```python
from build123d import *

# Parameters (mm, degrees)
F0_R      = 31.75
F1_DEPTH  = 101.6
F0_W      = 88.9
F0_H      = 6.35
F2_R      = 6.35
F3_SIZE   = 3.175
F6_DEPTH  = 88.9
F7_R      = 5.08
F8_W      = 12.7
F8_H      = 25.4
F9_DEPTH  = 88.9
F10_R     = 6.35
F11_R     = 9.525
F12_DEPTH = 6.35
F13_R     = 6.35
F14_DEPTH = 38.1


with BuildPart() as f1:
    # F0 (on Front) → F1 (new body)
    with BuildSketch(Plane.XZ):
        with Locations((0, 44.45)):
            Circle(F0_R)
    extrude(amount=-F1_DEPTH)

    # F2
    f2_edges = [f1.edges().sort_by_distance(p)[0] for p in [
        (-31.75, 0, 44.45),
        (-31.75, 101.6, 44.45),
    ]]
    fillet(f2_edges, radius=F2_R)

    # F5 (on offset) → F6 (join)
    with BuildSketch(Plane(origin=(0, 95.25, 0), x_dir=(-1, 0, 0), z_dir=(0, 1, 0))):
        Polygon((1.5875, 49.3358226153), (1.5875, 82.55), (-1.5875, 82.55), (-1.5875, 49.3358226153), (0, 47.1508163165), align=None)
        Polygon((21.1103036338, 76.2066565737), (1.5875, 49.3358226153), (1.5875, 46.6350062987), (4.1561289571, 47.4696044392), (23.6789325909, 74.3404383977), align=None)
        Polygon((1.5875, 46.6350062987), (1.5875, 49.3358226153), (0, 47.1508163165), (0.6063710429, 46.316218176), align=None)
        Polygon((0, 47.1508163165), (-1.5875, 49.3358226153), (-1.5875, 46.6350062987), (-0.6063710429, 46.316218176), align=None)
        Polygon((-1.5875, 46.6350062987), (-1.5875, 49.3358226153), (-21.1103036338, 76.2066565737), (-23.6789325909, 74.3404383977), (-4.1561289571, 47.4696044392), align=None)
        Polygon((4.1561289571, 47.4696044392), (1.5875, 46.6350062987), (1.5875, 45.6033862632), (2.5686289571, 45.2845981405), align=None)
        Polygon((-1.5875, 45.6033862632), (-1.5875, 46.6350062987), (-4.1561289571, 47.4696044392), (-2.5686289571, 45.2845981405), align=None)
        Polygon((35.7446887923, 57.7333497053), (4.1561289571, 47.4696044392), (2.5686289571, 45.2845981405), (5.1372579143, 44.45), (36.7258177494, 54.7137452661), align=None)
        Polygon((-2.5686289571, 45.2845981405), (-4.1561289571, 47.4696044392), (-35.7446887923, 57.7333497053), (-36.7258177494, 54.7137452661), (-5.1372579143, 44.45), align=None)
        Polygon((5.1372579143, 44.45), (2.5686289571, 45.2845981405), (1.9622579143, 44.45), (2.5686289571, 43.6154018595), align=None)
        Polygon((-1.9622579143, 44.45), (-2.5686289571, 45.2845981405), (-5.1372579143, 44.45), (-2.5686289571, 43.6154018595), align=None)
        Polygon((36.7258177494, 34.1862547339), (5.1372579143, 44.45), (2.5686289571, 43.6154018595), (4.1561289571, 41.4303955608), (35.7446887923, 31.1666502947), align=None)
        Polygon((-2.5686289571, 43.6154018595), (-5.1372579143, 44.45), (-36.7258177494, 34.1862547339), (-35.7446887923, 31.1666502947), (-4.1561289571, 41.4303955608), align=None)
        Polygon((2.5686289571, 43.6154018595), (1.5875, 43.2966137368), (1.5875, 42.2649937013), (4.1561289571, 41.4303955608), align=None)
        Polygon((-1.5875, 42.2649937013), (-1.5875, 43.2966137368), (-2.5686289571, 43.6154018595), (-4.1561289571, 41.4303955608), align=None)
        Polygon((4.1561289571, 41.4303955608), (1.5875, 42.2649937013), (1.5875, 39.5641773847), (21.1103036338, 12.6933434263), (23.6789325909, 14.5595616023), align=None)
        Polygon((1.5875, 39.5641773847), (1.5875, 42.2649937013), (0.6063710429, 42.583781824), (0, 41.7491836835), align=None)
        Polygon((-0.6063710429, 42.583781824), (-1.5875, 42.2649937013), (-1.5875, 39.5641773847), (0, 41.7491836835), align=None)
        Polygon((-1.5875, 39.5641773847), (-1.5875, 42.2649937013), (-4.1561289571, 41.4303955608), (-23.6789325909, 14.5595616023), (-21.1103036338, 12.6933434263), align=None)
        Polygon((1.5875, 6.35), (1.5875, 39.5641773847), (0, 41.7491836835), (-1.5875, 39.5641773847), (-1.5875, 6.35), align=None)
    extrude(amount=-F6_DEPTH)

    # F7
    f7_edges = [f1.edges().sort_by_distance(p)[0] for p in [
        (0, 95.25, 82.55),
        (-22.394618, 95.25, 75.273547),
        (22.394618, 95.25, 75.273547),
        (36.235253, 95.25, 56.223547),
        (36.235253, 95.25, 32.676453),
        (22.394618, 95.25, 13.626453),
        (0, 95.25, 6.35),
        (-22.394618, 95.25, 13.626453),
        (-36.235253, 95.25, 32.676453),
        (-36.235253, 95.25, 56.223547),
        (-36.235253, 6.35, 56.223547),
        (-36.235253, 6.35, 32.676453),
        (-22.394618, 6.35, 75.273547),
        (0, 6.35, 82.55),
        (22.394618, 6.35, 75.273547),
        (36.235253, 6.35, 56.223547),
        (36.235253, 6.35, 32.676453),
        (22.394618, 6.35, 13.626453),
        (0, 6.35, 6.35),
        (-22.394618, 6.35, 13.626453),
    ]]
    fillet(f7_edges, radius=F7_R)



with BuildPart() as f1b:
    # F0 (on Front) → F1, piece 2 (new body)
    with BuildSketch(Plane.XZ):
        Rectangle(F0_W, F0_H)
    extrude(amount=-F1_DEPTH)

    # F3
    f3_edges = [f1b.edges().sort_by_distance(p)[0] for p in [
        (0, 0, 3.175),
        (44.45, 50.8, 3.175),
        (-44.45, 50.8, 3.175),
        (0, 101.6, 3.175),
    ]]
    chamfer(f3_edges, length=F3_SIZE)


with BuildPart() as f1_1:
    add(f1.part)

    add(f1b.part)  # F9 merges F1b
    # F8 (on offset) → F9 (join)
    with BuildSketch(Plane(origin=(0, 95.25, 0), x_dir=(-1, 0, 0), z_dir=(0, 1, 0))):
        with Locations((6.35, 12.7)):
            Rectangle(F8_W, F8_H)
        with Locations((-6.35, 12.7)):
            Rectangle(F8_W, F8_H)
    extrude(amount=-F9_DEPTH)

    # F10
    f10_edges = [f1_1.edges().sort_by_distance(p)[0] for p in [
        (-44.45, 101.6, -1.5875),
        (44.45, 101.6, -1.5875),
        (44.45, 0, -1.5875),
        (-44.45, 0, -1.5875),
    ]]
    fillet(f10_edges, radius=F10_R)

    # F11 (on face) → F12 (join)
    with BuildSketch(Plane.XZ):
        with Locations((0, 44.45)):
            Circle(F11_R)
    extrude(amount=F12_DEPTH)

    # F13 (on face) → F14 (join)
    with BuildSketch(Plane.XZ.offset(6.35)):
        with Locations((0, 44.45)):
            Circle(F13_R)
    extrude(amount=F14_DEPTH)


solid = f1_1.part
```
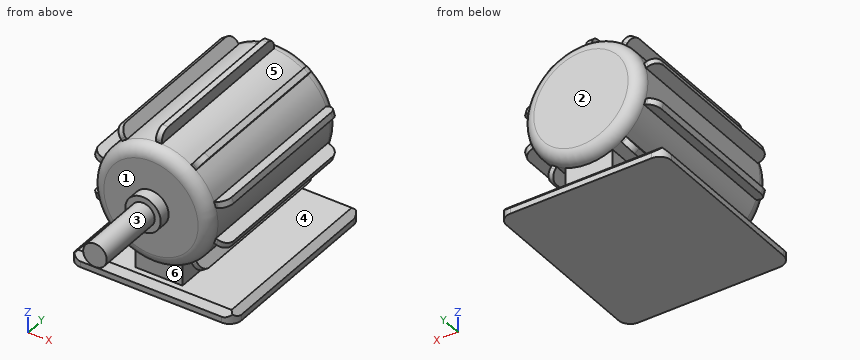
Work out the finished part from the listing and answer in its coordinate system (mm). Face numbers are marked on the shaded views. A direction names the side the tool comes from. Give positions to 0.01 mm unless a question says otherwise; leave off trailing zeros. Write each loop counter-clockwise with the first axis right and the second up, starting at its lowest first coordinate (ties: lowest second). Pieces come first, ordered by that corner, then holes. Notation, with made-up numbers: (86.5, 3) -> (108.5, 3) arc R30 ccw to (108.5, 37) -> close; hole circle Ø6 at (-8, 24.25). An arc over 180 degrees is marked (long way). Write item = value, one per line.
Q1. Section A-A on x = 0 is taken. Determine the outline of the cut face in (y, z) (3 decimals).
Computed values:
outline = (-44.45, 38.1) -> (-6.35, 38.1) -> (-6.35, 34.925) -> (0, 34.925) -> (0, 19.05) arc R6.35 ccw to (6.35, 12.7) -> (6.35, 3.175) -> (3.175, 3.175) -> (0, 0) -> (0, -3.175) -> (101.6, -3.175) -> (101.6, 0) -> (98.425, 3.175) -> (95.25, 3.175) -> (95.25, 12.7) arc R6.35 ccw to (101.6, 19.05) -> (101.6, 69.85) arc R6.35 ccw to (95.25, 76.2) -> (95.25, 77.47) arc R5.08 ccw to (90.17, 82.55) -> (11.43, 82.55) arc R5.08 ccw to (6.35, 77.47) -> (6.35, 76.2) arc R6.35 ccw to (0, 69.85) -> (0, 53.975) -> (-6.35, 53.975) -> (-6.35, 50.8) -> (-44.45, 50.8) -> close
Q2. Flat-ended cylindrical pins translate along their axes: pin 1 Ø3.5 at (y, z) = (45.5, 11) entering from -X; pin 2 Ø1.9 at (y, z) = (55, 80) entering from +X; pin 3 Ø13.5 at (x, z) = (4, 11) entering from -Y; pin 4 Ø10 at (x, z) = (19.5, 63) entering from +Y. Find the tip coordinate at first contact, or state that the pin passes through.
Computed values:
pin_1 = -21.19
pin_2 = 1.59
pin_3 = 0.19
pin_4 = 101.6
Q3. Section B-B on z = 44.45 is taken. Determine the outline of the cut face in (x, y) (3 decimals).
Computed values:
outline = (-31.75, 6.35) arc R6.35 ccw to (-25.4, 0) -> (-9.525, 0) -> (-9.525, -6.35) -> (-6.35, -6.35) -> (-6.35, -44.45) -> (6.35, -44.45) -> (6.35, -6.35) -> (9.525, -6.35) -> (9.525, 0) -> (25.4, 0) arc R6.35 ccw to (31.75, 6.35) -> (31.75, 95.25) arc R6.35 ccw to (25.4, 101.6) -> (-25.4, 101.6) arc R6.35 ccw to (-31.75, 95.25) -> close
Q4. A tool of negligible diameter and unlimited length cuts with its end or side. For the marked faces 1 and 2, from which of +Z, -Z, +X, -X, +Y, -Y can it reach the whole face along a straight path? Write none if from no direction.
Computed values:
face_1 = -Y
face_2 = +Z, -Z, +X, -X, +Y
Q5. Consider line 1 along X through (y, z) = (17.5, 72); line 2 along Y through (x, z) = (13, 46.5); line 3 along Z through (x, y) = (-18, 66.5) (3 decimals). Determine where each line is inside the solid, lowest interval first.
Computed values:
line_1 = -21.98 to -18.05, -15.78 to 15.78, 18.05 to 21.98
line_2 = 0 to 101.6
line_3 = -3.175 to 3.175, 16.974 to 71.926
Q6. Section C-C on y = -13.5 is taken. Determine the outline of the cut face in (x, z), and give its area (3 significant figures).
Computed values:
outline = circle Ø12.7 at (0, 44.45)
area = 127 mm^2
Q7. For a pull along Z with two mould halves and no side action, classify the marked faces 3, 4, 5 and 6 as pulls with the +Z half, pulls with the -Z half, needs draft (parallel to the pull), parting line crosses it, or undercut.
Computed values:
face_3 = parting line crosses it
face_4 = undercut
face_5 = pulls with the +Z half
face_6 = undercut
